Drawing for the job (mm, zero at the part's lowest x, y, z). A direction names the side the tool comes from. Coordinates: 2 decimals unless noted, no trailing zeros. Write each loop counter-clockwise with the first axis right and the second up, starting at its lowest first coordinate (ties: lowest second). Pieces come first, ordered by that corner, then holes.
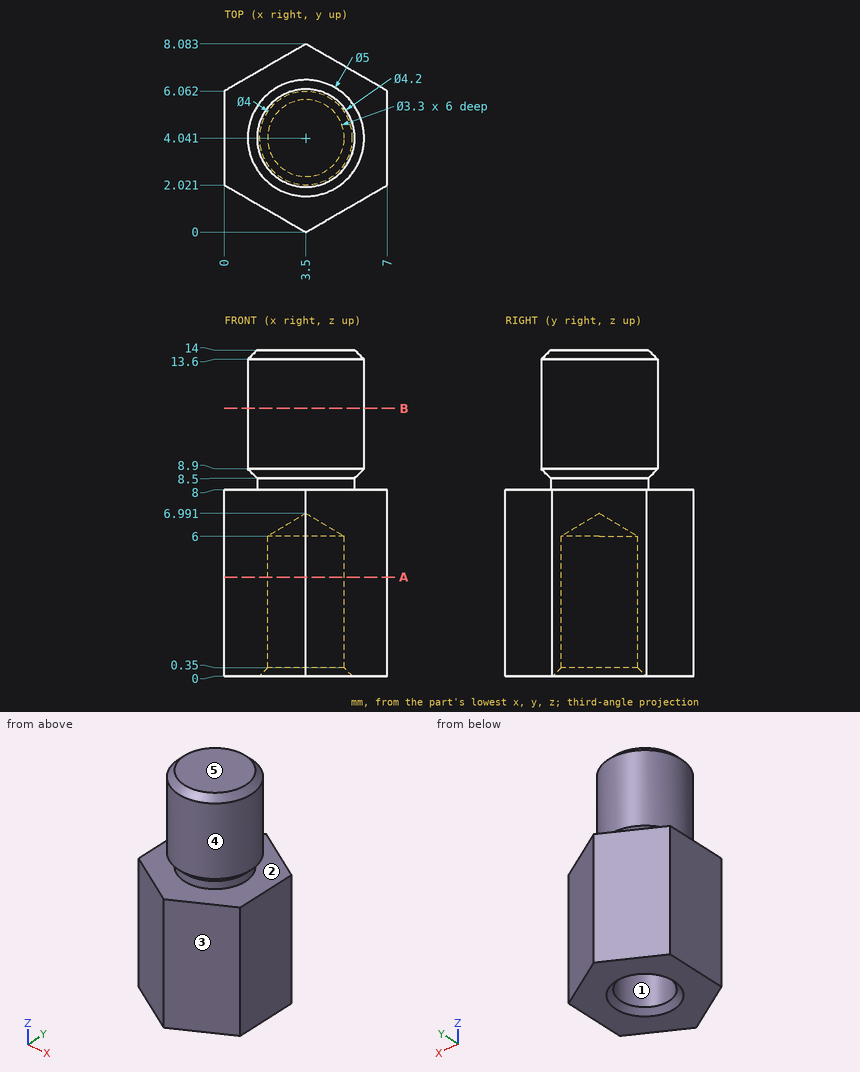
Item 1: Wall check: line 1 along Z through (x, y) = (4.5, 6.75); line 2 along Y through (x, z) = (3.5, 10.25); line 3 along X through (y, z) = (4.25, 4.25). Give the ranges that are in metal, low to high.
Item 2: Which spindle directions (+Z, -Z, +X, -X, +Y, -Y) get a long thin tool onto all of the face, cutting with end or side? Do the marked faces 4 and 5. Say none if no direction does.
Item 3: Flat gauge pins, fed straight in: pin 1 Ø3 at (y, z) = (4.5, 4) entering from -X; pin 2 Ø2 at (y, z) = (3, 10) entering from -X; pin 3 Ø2 at (x, y) = (3, 4) entering from -Z. Where does each tip first touch, or does it go through?
Item 4: Saw through at A-A, the plane z = 4.25. Write the cut outline in (x, y).
Item 5: Two-plate mould, pull along Y, no slides. Class the marked faces 1, 2 and 3: +Y half, -Y half, draft (parallel to the pull), parting line (faces both ways), or undercut.
Item 6: Saw through at B-B, the plane z = 11.5. Write the cut outline in (x, y), and give its area (3 significant figures).
Working result:
1. line 1: z = 0 to 8
1. line 2: y = 1.54 to 6.54
1. line 3: x = 0 to 1.86, 5.14 to 7
2. face 4: +Z
2. face 5: +Z, +X, -X, +Y, -Y
3. pin 1: stops at x = 0
3. pin 2: stops at x = 1
3. pin 3: stops at z = 6.09
4. outline: (0, 2.02) - (3.5, 0) - (7, 2.02) - (7, 6.06) - (3.5, 8.08) - (0, 6.06) - close; hole circle Ø3.3 at (3.5, 4.04)
5. face 1: undercut
5. face 2: draft
5. face 3: -Y half
6. outline: circle Ø5 at (3.5, 4.04)
6. area: 19.6 mm2
